The model under review builds one solid part; all positions refer to its coordinate system, in mm. A direction names the side the tool comes from. Round coordinates to 2 decimals unless told otherwise and drop trailing zeros. Order: outer loops, then holes, each group sorted by start corner. A loop starts at its lowest first (then second) coordinate and runs counter-clockwise, first axis right, second up. Notation, with made-up numbers: (77, -20) - (102, -20) arc R8 ccw to (102, -16) - close; hole circle Ø11 at (-38, 5.5). An arc over 180 degrees is marked (long way). One line per question, with ' | ' between items. Start each with the question number.
Item 1: Tool access review of faces 4 (the face through (-0.76, -18.53, 0.14)), 5 (the face through (16, 8.5, 0)), 6 (the face through (-0.806, 18.539, 0.14)): name each direction out of +Z, -Z, +X, -X, +Y, -Y from which nothing blocks a thin tool from reaching the whole face with its end or side.
Item 2: Add section B-B on x = 10. State the section outline as (y, z) points, and give its area (3 significant figures).
Item 3: Insertion check: pin 1 Ø3.5 at (x, z) = (17, 2) entering from +Y; pin 2 Ø1 at (x, z) = (-17, 3.5) entering from +Y; pin 3 Ø5 at (y, z) = (-15, 3.5) entering from -X; pin 4 Ø2 at (y, z) = (-3.5, 4) entering from -X. Each pin has a flat end and moves straight along its axis. Give the tip position at first contact, or say it passes through.
Item 4: Draft analysis for pull direction X (two halves, no side actions). For faces 1 (the face through (0.906, 18.497, 0.14)), 2 (the face through (-19.894, -5.543, 0.14)), 3 (the face through (14.74, -14.47, 0.14)), state which applies: +X half, -X half, draft (parallel to the pull), parting line (faces both ways), or undercut.
Item 5: Add section C-C on y = -9.5. State the section outline as (x, z) points, and give its area (3 significant figures).
Item 6: For L1, parallel to Y at x = -15, z = 6.75; L2, parallel to Y at x = 12, z = 9.25; L3, parallel to X at y = 17, z = -7.25, list the stretches that pass through material, from the lowest coordinate up. Write a range as [from, to].
from build123d import *

# Parameters (mm, degrees)
EXTRUDE_1_DEPTH          = 10
CUT_EXTRUDE_1_DEPTH      = 20
PATTERN_CIRCULAR_1_COUNT = 6
SKETCH_3_R               = 3
CUT_EXTRUDE_2_DEPTH      = 20
PATTERN_CIRCULAR_2_COUNT = 6


with BuildPart() as part:
    # 草图1 → 凸台-拉伸1 (new, symmetric)
    with BuildSketch(Plane.XY):
        Polygon((23.094010768, 0), (11.547005384, 20), (-11.547005384, 20), (-23.094010768, 0), (-11.547005384, -20), (11.547005384, -20), align=None)
    extrude(amount=EXTRUDE_1_DEPTH, both=True)

    # 草图2 → 切除-拉伸1 (cut)
    with BuildSketch(Plane.XY.offset(10)):
        Polygon((-14.722431864, 8.5), (-17.320508076, 13), (-19.918584287, 8.5), align=None)
    cut_extrude_1 = extrude(amount=-CUT_EXTRUDE_1_DEPTH, mode=Mode.SUBTRACT)

    # 阵列(圆周)1: 切除-拉伸1 ×6 about axis
    pattern_circular_1_axis = Axis((0.061936572, -0.035759097, 0), (0, 0, 1))
    for i in range(1, PATTERN_CIRCULAR_1_COUNT):
        add(cut_extrude_1.rotate(pattern_circular_1_axis, i * 360 / PATTERN_CIRCULAR_1_COUNT), mode=Mode.SUBTRACT)

    # 草图3 → 切除-拉伸2 (cut)
    with BuildSketch(Plane.XY.offset(10)):
        with Locations((-23.094010768, 0)):
            Circle(SKETCH_3_R)
    cut_extrude_2 = extrude(amount=-CUT_EXTRUDE_2_DEPTH, mode=Mode.SUBTRACT)

    # 阵列(圆周)2: 切除-拉伸2 ×6 about axis
    pattern_circular_2_axis = Axis((0.158034709, -0.00459912, 0), (0, 0, 1))
    for i in range(1, PATTERN_CIRCULAR_2_COUNT):
        add(cut_extrude_2.rotate(pattern_circular_2_axis, i * 360 / PATTERN_CIRCULAR_2_COUNT), mode=Mode.SUBTRACT)


solid = part.part
Determined:
1) face 4: +Z, -Z, -Y | face 5: +Z, -Z, +X | face 6: +Z, -Z, +Y
2) outline: (-17.73, -10) - (17.72, -10) - (17.72, 10) - (-17.73, 10) - close | area: 709 mm2
3) pin 1: y = 13.59 | pin 2: y = 8.5 | pin 3: x = -15.88 | pin 4: x = -21.59
4) face 1: undercut | face 2: -X half | face 3: +X half
5) outline: (-15.26, -10) - (15.38, -10) - (15.38, 10) - (-15.26, 10) - close | area: 613 mm2
6) L1: [-14.02, -9.05], [-8.57, 8.5], [8.98, 14.02] | L2: [-17.15, 17.14] | L3: [-13.28, 13.28]
